Autodesk Inventor part; units mm, degrees
ref_plane "YZ Plane" through (0, 0, 0) normal (1, 0, 0) x (0, 1, 0)
ref_plane "XZ Plane" through (0, 0, 0) normal (0, 1, 0) x (-1, 0, 0)
ref_plane "XY Plane" through (0, 0, 0) normal (0, 0, 1) x (1, 0, 0)
sketch "Sketch1" plane through (0, 0, 0) normal (0, 0, 1) x (1, 0, 0)
  circle A0 centre (0, 0) radius 37.5
  circle A1 centre (0, 0) radius 12.5
  dimension "d15" = 25
  dimension "d16" = 75
extrude "Plate1" add sketch "Sketch1" along normal blind 3
sketch "Sketch2" plane through (0, 0, 0) normal (0, 0, -1) x (-1, 0, 0)
  line L0 (-27.3167, 25.2399) -> (172.6833, 25.2399) construction
  line L1 (172.6833, 25.2399) -> (172.6833, 5.2399) construction
  line L2 (172.6833, 5.2399) -> (-27.3167, 5.2399) construction
  line L3 (-27.3167, 5.2399) -> (-27.3167, 25.2399) construction
  point P0 (0, 0)
  point P1 (-251, -525)
  dimension "d6" = 200
  dimension "d9" = 20
mark "Mark1"
sketch "Sketch3" plane through (0, 0, 3) normal (0, 0, 1) x (1, 0, 0)
  circle A0 centre (0, 0) radius 12.5 construction
  circle A1 centre (0, 0) radius 37.5 construction
  circle A2 centre (0, 30) radius 3
  line L0 (0, 37.5) -> (0, 12.5) construction
  circle A3 centre (0, 0) radius 30 construction
  dimension "d26" = 60
  dimension "d17" = 6
  dimension "d19" = 7.5
extrude "Cut1" cut sketch "Sketch3" against normal blind 3
pattern_circular "Circular Pattern1" count 4 over 360 about axis through (0, 0, 0) along (0, 0, 1) of "Cut1"
equation "\"d20\" = Thickness"
equation "\"d2\" = Thickness"
equation "\"BendReliefWidth\" = Thickness"
equation "\"BendReliefDepth\" = 0.5 * Thickness"
equation "\"CornerReliefSize\" = 4 * Thickness"
equation "\"MinimumRemnant\" = 2 * Thickness"
equation "\"TransitionRadius\" = BendRadius"
equation "\"JacobiRadiusSize\" = BendRadius"
equation "\"GapSize\" = Thickness"
properties part number "TRM 029 coupling ring" material "AISI 304"
Design review of the part built by this model. Coordinates are the model's own, in mm. Coordinates: 2 decimals unless noted, no trailing zeros. Write each loop counter-clockwise with the first axis right and the second up, starting at its lowest first coordinate (ties: lowest second). Pieces come first, ordered by that corner, then holes.
1) Mouldability with a two-part tool opening along Y and no side actions: class faces 1 (the cylindrical face through (32.03, 2.21, 1.52)), 2 (the cylindrical face through (11.923, -3.755, 1.479)), 3 (the flat face through (-9, 9, 0)), 4 (the cylindrical face through (-4.88, -37.18, 1.48)) as +Y half, -Y half, draft (parallel to the pull), parting line (faces both ways), or undercut.
2) Add section C-C (z = 2). Write out the cut boundary in (x, y).
3) Add section A-A (x = 0). Write out the cut boundary in (y, z).
4) To check wall thickness, follow L1, parallel to Y at x = 0, z = 1.3; L2, parallel to X at y = 0.5, z = 0.3; L3, parallel to X at y = -30, z = 1.65. State the ranges of each line that lie inside material, in increasing order.
5) Add section D-D (x = 30). Write out the cut boundary in (y, z).
6) Insertion check: pin 1 (22.5 mm diameter, centred on x = 0, y = 0, fed in from +Z); pin 2 (1.5 mm diameter, centred on x = 23.5, z = 0.5, fed in from -Y); pin 3 (1 mm diameter, centred on x = -13, z = 1, fed in from -Y); pin 4 (1 mm diameter, centred on x = 9.5, z = 0.5, fed in from +Y). Each pin has a flat end and moves straight along its axis. Give the tip position at first contact, or say it passes through.
Check result:
1. face 1: undercut
1. face 2: undercut
1. face 3: draft
1. face 4: parting line
2. outline: circle Ø75 at (0, 0); hole circle Ø6 at (-30, 0); hole circle Ø25 at (0, 0); hole circle Ø6 at (0, -30); hole circle Ø6 at (0, 30); hole circle Ø6 at (30, 0)
3. outline: (-37.5, 0) - (-33, 0) - (-33, 3) - (-37.5, 3) - close; (-27, 0) - (-12.5, 0) - (-12.5, 3) - (-27, 3) - close; (12.5, 0) - (27, 0) - (27, 3) - (12.5, 3) - close; (33, 0) - (37.5, 0) - (37.5, 3) - (33, 3) - close
4. L1: y = -37.5 to -33, -27 to -12.5, 12.5 to 27, 33 to 37.5
4. L2: x = -37.5 to -32.96, -27.04 to -12.49, 12.49 to 27.04, 32.96 to 37.5
4. L3: x = -22.5 to -3, 3 to 22.5
5. outline: (-22.5, 0) - (-3, 0) - (-3, 3) - (-22.5, 3) - close; (3, 0) - (22.5, 0) - (22.5, 3) - (3, 3) - close
6. pin 1: passes through
6. pin 2: stops at y = -29.81
6. pin 3: stops at y = -35.36
6. pin 4: stops at y = 36.4
